Geometry check sheet. Reference: the model listing, model coordinates, mm. A direction names the side the tool comes from. Round coordinates to 2 decimals unless told otherwise and drop trailing zeros. Loops run counter-clockwise (first coordinate to the right, second up) from the corner with the lowest first, then second, coordinate; pieces in that order, holes last. Notation, with made-up numbers: (40, 71) -> (68, 71) arc R22 cw to (68, 82) -> close; hole circle Ø3 at (27, 4). An arc over 180 degrees is marked (long way). Use a Markdown table: item, result. Add a question column.
Q1. Sectioned sample at A-A, the plane y = 1. Enter the section's corners in (x, z) (3 decimals).
Q2. Set-up check for faces 1 (the face through (4, 0, 0)), 2 (the face through (-2.9, -1, 0)), 3 (the face through (0, 1, -2.925)): record each of +Z, -Z, +X, -X, +Y, -Y from which the full face is reachable in a straight line by a thin tool's end or side.
Q3. Sectioned sample at D-D, the plane z = -1.25. Enter the section's corners in (x, y), then the cut area to 3 significant figures.
Q4. Sectioned sample at C-C, the plane x = 0. Enter the section's corners in (y, z) (3 decimals), then the cut area to 3 significant figures.
Q5. Material ranges on L1, parallel to X at y = 1.25, z = 0; L2, parallel to Z at x = 0, y = -0.3 (3 decimals); L3, parallel to X at y = 2.15, z = 1.15, recorded low to high.
Q6. Gauge pin test, flat ends, axial feed: P1, Ø2, axis at x = 4.5, z = 1, coming from the -Y side; P2, Ø1.4, axis at y = -0.5, z = 1, coming from the +X side. Record the tip position at first contact, or that the pin passes through.
Q7. Sectioned sample at B-B, the plane z = 0. Enter the section's corners in (x, y), then the cut area to 3 significant figures.
Autodesk Inventor part; units mm, degrees
ref_plane "YZ Plane" through (0, 0, 0) normal (1, 0, 0) x (0, 1, 0)
ref_plane "XZ Plane" through (0, 0, 0) normal (0, 1, 0) x (-1, 0, 0)
ref_plane "XY Plane" through (0, 0, 0) normal (0, 0, 1) x (1, 0, 0)
sketch "Esquisse1" plane through (0, 0, 0) normal (0, 0, 1) x (1, 0, 0)
  line L0 (-5.65, 0) -> (5.65, 0)
  line L1 (5.65, 0) -> (5.65, 1.75)
  line L2 (5.65, 1.75) -> (4.125, 2.8)
  line L3 (4.125, 2.8) -> (-4.125, 2.8)
  line L4 (-4.125, 2.8) -> (-5.65, 1.75)
  line L5 (-5.65, 1.75) -> (-5.65, 0)
  point P0 (0, 0)
  dimension "d0" = 11.3
  dimension "d1" = 2.8
  dimension "d2" = 8.25
  dimension "d3" = 5.65
  dimension "d4" = 1.75
extrude "Extrusion1" add sketch "Esquisse1" along normal mid plane 5.85
sketch "Esquisse2" plane through (-5.65, 0, 2.925) normal (0, -1, 0) x (1, 0, 0)
  line L0 (2.75, -5.85) -> (8.55, -5.85)
  line L1 (8.55, -5.85) -> (8.55, 0)
  line L2 (8.55, 0) -> (2.75, 0)
  line L3 (2.75, 0) -> (2.75, -5.85)
  line L4 (2.75, -5.85) -> (8.55, 0) construction
  line L5 (8.55, -5.85) -> (2.75, 0) construction
  line L6 (0, 0) -> (11.3, 0)
  point P0 (5.65, -2.925)
  dimension "d7" = 5.8
extrude "Extrusion2" add sketch "Esquisse2" along normal blind 1.3
sketch "Esquisse3" plane through (-4.125, 2.8, 2.925) normal (0, 1, 0) x (1, 0, 0)
  point P0 (4.125, 2.925)
  point P1 (4.125, 2.925)
hole "Perçage1" at (0, 2.8, 0) direction (0, -1, 0) diameter 3.242 depth 11.8 tip angle 118
fillet "Congé1" radius 0.5 2 edges at (-5.65, 1.75, 0) (5.65, 1.75, 0)
fillet "Congé2" radius 0.75 2 edges at (4.125, 2.8, 0) (-4.125, 2.8, 0)
fillet "Congé3" radius 0.5 18 edges at (-5.5926, 1.7198, 2.925) (-5.65, 0.7436, 2.925) (-4.1145, 2.7662, 2.925) (0, 2.8, 2.925) (4.1145, 2.7662, 2.925) (4.8753, 2.2834, 2.925) (5.5926, 1.7198, 2.925) (5.65, 0.7436, 2.925) (-4.8753, 2.2834, 2.925) (-4.1145, 2.7662, -2.925) (0, 2.8, -2.925) (4.1145, 2.7662, -2.925) (4.8753, 2.2834, -2.925) (5.5926, 1.7198, -2.925) (5.65, 0.7436, -2.925) (-5.5926, 1.7198, -2.925) (-5.65, 0.7436, -2.925) (-4.8753, 2.2834, -2.925)
properties part number "Noix M4" material "Acier"
Values:
| question | item | result |
|---|---|---|
| 1 | outline | (-5.65, -2.425) arc R0.5 ccw to (-5.15, -2.925) -> (5.15, -2.925) arc R0.5 ccw to (5.65, -2.425) -> (5.65, 2.425) arc R0.5 ccw to (5.15, 2.925) -> (-5.15, 2.925) arc R0.5 ccw to (-5.65, 2.425) -> close; hole circle Ø3.242 at (0, 0) |
| 2 | face 1 | +Z, -Z, +X, -Y |
| 2 | face 2 | +Z, -Z, -X, -Y |
| 2 | face 3 | -Z, +X, -X, +Y, -Y |
| 3 | outline | (-5.65, 0) -> (-2.9, 0) -> (-2.9, -1.3) -> (-1.03, -1.3) -> (-1.03, 2.8) -> (-3.89, 2.8) arc R0.75 ccw to (-4.32, 2.67) -> (-5.43, 1.9) arc R0.5 ccw to (-5.65, 1.49) -> close; (1.03, -1.3) -> (2.9, -1.3) -> (2.9, 0) -> (5.65, 0) -> (5.65, 1.49) arc R0.5 ccw to (5.43, 1.9) -> (4.32, 2.67) arc R0.75 ccw to (3.89, 2.8) -> (1.03, 2.8) -> close |
| 3 | area | 29.1 mm^2 |
| 4 | outline | (-1.3, -2.925) -> (2.3, -2.925) arc R0.5 ccw to (2.8, -2.425) -> (2.8, -1.621) -> (-1.3, -1.621) -> close; (-1.3, 1.621) -> (2.8, 1.621) -> (2.8, 2.425) arc R0.5 ccw to (2.3, 2.925) -> (-1.3, 2.925) -> close |
| 4 | area | 10.6 mm^2 |
| 5 | L1 | -5.65 to -1.62, 1.62 to 5.65 |
| 5 | L2 | -2.925 to -1.621, 1.621 to 2.925 |
| 5 | L3 | -5.07 to -1.14, 1.14 to 5.07 |
| 6 | P1 | y = 0 |
| 6 | P2 | x = 5.65 |
| 7 | outline | (-5.65, 0) -> (-2.9, 0) -> (-2.9, -1.3) -> (-1.62, -1.3) -> (-1.62, 2.8) -> (-3.89, 2.8) arc R0.75 ccw to (-4.32, 2.67) -> (-5.43, 1.9) arc R0.5 ccw to (-5.65, 1.49) -> close; (1.62, -1.3) -> (2.9, -1.3) -> (2.9, 0) -> (5.65, 0) -> (5.65, 1.49) arc R0.5 ccw to (5.43, 1.9) -> (4.32, 2.67) arc R0.75 ccw to (3.89, 2.8) -> (1.62, 2.8) -> close |
| 7 | area | 24.3 mm^2 |
